Job drawing, mm, ordinate dimensions from the low corner. One solid piece. A direction names the side the tool comes from. Round coordinates to 2 decimals unless told otherwise and drop trailing zeros. Loops run counter-clockwise (first coordinate to the right, second up) from the corner with the lowest first, then second, coordinate; pieces in that order, holes last. Notation, with made-up numbers: M 33.5,-25.75 L 41.5,-25.75 A10 cw 41.5,-19.75 Z; hole C 62.25,-33 d4. An arc over 180 degrees is marked long. Use one line per item in the form item = value. Start each with the question number.
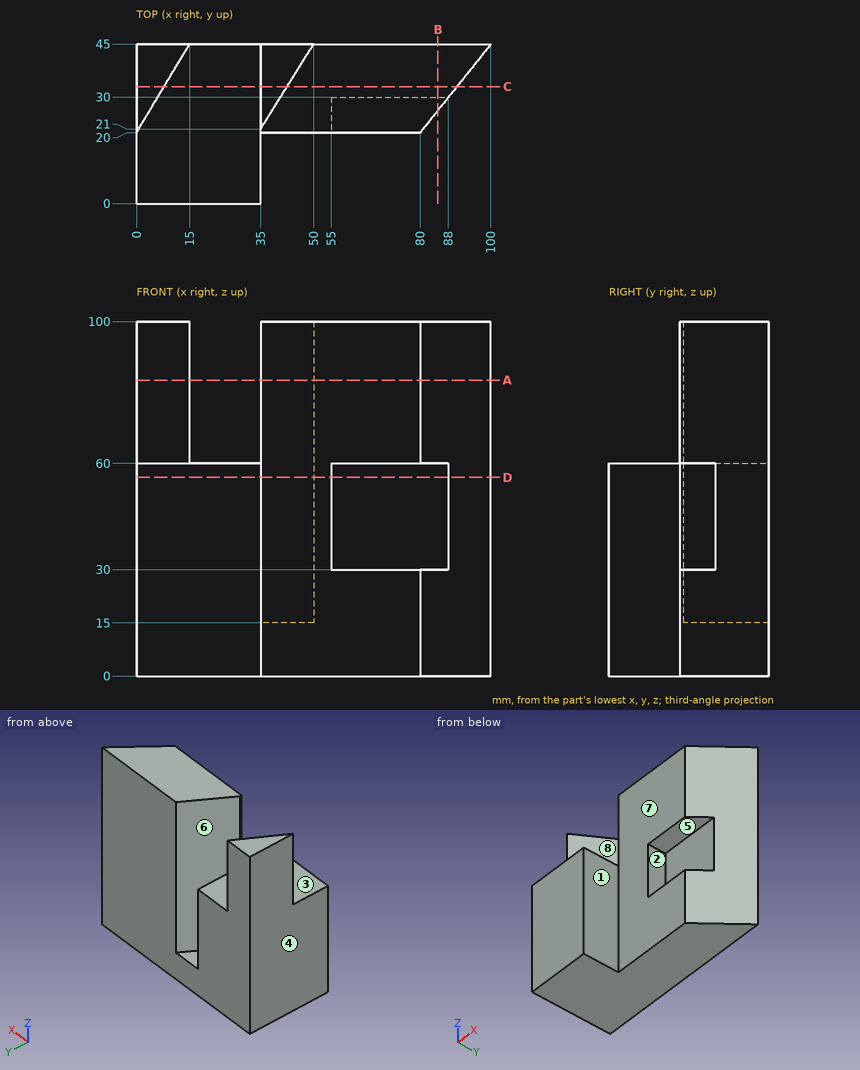
Q1. Saw through at D-D (z = 56). Give the cut face in (x, y), and give its area (3 significant figures).
Q2. Wall check: probe 1 along Z at (x, y) = (58, 24); probe 2 along Y at (x, z) = (53, 89); probe 3 along X at (y, z) = (29.5, 65.5). Give the ranges that are in metal, low to high.
Q3. Drop flat-ended pins along their axis: P1, Ø13.5, axis at x = 47.5, z = 53, coming from the -Y side; P2, Ø24, axis at x = 77.5, z = 45, coming from the -Y side; P3, Ø10, axis at y = 7, z = 19.5, coming from the +X side; P4, Ø10, axis at y = 14, z = 70.5, coming from the -X side. Give the stop position or say it passes through.
Q4. Saw through at A-A (z = 83.5). Give the cut face in (x, y).
Q5. Pull direction Z, two halves, no side cores. Call the marked faces 1, 2 and 3: pulls with the +Z half, pulls with the -Z half, needs draft (parallel to the pull), parting line crosses it, or undercut.
Q6. Saw through at C-C (y = 33). Give the cut face in (x, z).
Q7. Tool access for the marked faces 4, 5, 6, 7 and 8: list every direction of +Z, -Z, +X, -X, +Y, -Y with a clear straight run to the whole face (end or side of a thin tool).
Q8. Saw through at B-B (x = 85). Give the cut face in (y, z).
Filled in:
q1.outline = M 0,0 L 35,0 L 35,20 L 55,20 L 55,30 L 88,30 L 100,45 L 50,45 L 35,21 L 35,45 L 0,45 Z
q1.area = 2,480 mm²
q2.probe_1 = 0 to 30, 60 to 100
q2.probe_2 = 20 to 45
q2.probe_3 = 0 to 5.7, 40.31 to 87.6
q3.P1 = 20
q3.P2 = 30
q3.P3 = 35
q3.P4 = through
q4.outline = M 0,20 L 15,45 L 0,45 Z; M 35,20 L 80,20 L 100,45 L 50,45 L 35,21 Z
q5.face_1 = needs draft
q5.face_2 = undercut
q5.face_3 = pulls with the +Z half
q6.outline = M 0,0 L 90.4,0 L 90.4,100 L 42.5,100 L 42.5,15 L 35,15 L 35,60 L 7.8,60 L 7.8,100 L 0,100 Z
q7.face_4 = +Z, -Z, -X, +Y, -Y
q7.face_5 = +X, -Y
q7.face_6 = +Z, +Y
q7.face_7 = +Z, -Z, +X, -Y
q7.face_8 = +Z, -Y
q8.outline = M 26.25,0 L 45,0 L 45,100 L 26.25,100 L 26.25,60 L 30,60 L 30,30 L 26.25,30 Z
